```python
from build123d import *

# Parameters (mm, degrees)
BOSS_EXTRUDE3_DEPTH = 37
SKETCH7_OUTSIDE_W   = 24.466
SKETCH7_OUTSIDE_H   = 49.466
CUT_EXTRUDE4_DEPTH  = 37
SKETCH8_R           = 1.5
CUT_EXTRUDE5_DEPTH  = 3.5
SKETCH9_R           = 1.5
CUT_EXTRUDE6_DEPTH  = 3.5
SKETCH10_R          = 1.4
BOSS_EXTRUDE4_DEPTH = 3


with BuildPart() as part:
    # Sketch1 → Boss-Extrude3 (new body)
    with BuildSketch(Plane(origin=(0, 0, 0), x_dir=(1, 0, 0), z_dir=(0, 1, 0))):
        Polygon((-15.830224571, 22.390751722), (-15.830224571, -12.609248278), (-3.830224571, -12.609248278), (-3.830224571, -6.609248278), (-9.830224571, -6.609248278), (-9.830224571, 22.390751722), align=None)
    extrude(amount=BOSS_EXTRUDE3_DEPTH)

    # Sketch7 outside → Cut-Extrude4 (cut)
    with BuildSketch(Plane(origin=(0, 0, -22.390751722), x_dir=(-1, 0, 0), z_dir=(0, 0, -1))):
        with Locations((9.83, 18.5)):
            Rectangle(SKETCH7_OUTSIDE_W, SKETCH7_OUTSIDE_H)
        with BuildLine():
            Line((12.830224571, 37), (-5.541662032, 37))
            Line((-5.541662032, 37), (-5.541662032, 0))
            Line((-5.541662032, 0), (12.830224571, 0))
            ThreePointArc((12.830224571, 0), (14.951544915, 0.878679656), (15.830224571, 3))
            Line((15.830224571, 3), (15.830224571, 34))
            ThreePointArc((15.830224571, 34), (14.951544915, 36.121320344), (12.830224571, 37))
        make_face(mode=Mode.SUBTRACT)
    extrude(amount=-CUT_EXTRUDE4_DEPTH, mode=Mode.SUBTRACT)

    # Sketch8 → Cut-Extrude5 (cut)
    with BuildSketch(Plane(origin=(-9.830224571, 0, 0), x_dir=(0, 0, -1), z_dir=(1, 0, 0))):
        with Locations((-0.109248278, 34)):
            Circle(SKETCH8_R)
        with Locations((8.890751722, 34)):
            Circle(SKETCH8_R)
        with Locations((-0.109248278, 3)):
            Circle(SKETCH8_R)
        with Locations((8.890751722, 3)):
            Circle(SKETCH8_R)
        with Locations((17.890751722, 3)):
            Circle(SKETCH8_R)
        with Locations((17.890751722, 34)):
            Circle(SKETCH8_R)
    extrude(amount=-CUT_EXTRUDE5_DEPTH, mode=Mode.SUBTRACT)

    # Sketch9 → Cut-Extrude6 (cut)
    with BuildSketch(Plane(origin=(0, 0, 6.609248278), x_dir=(-1, 0, 0), z_dir=(0, 0, -1))):
        with Locations((6.830224571, 34)):
            Circle(SKETCH9_R)
        with Locations((6.830224571, 3)):
            Circle(SKETCH9_R)
    extrude(amount=-CUT_EXTRUDE6_DEPTH, mode=Mode.SUBTRACT)

    # Sketch10 → Boss-Extrude4 (add)
    with BuildSketch(Plane(origin=(-9.830224571, 0, 0), x_dir=(0, 0, -1), z_dir=(1, 0, 0))):
        with Locations(Location((4.390751722, 3, 0), (0, 0, 180))):
            Circle(SKETCH10_R)
        with Locations(Location((4.390751722, 34, 0), (0, 0, 180))):
            Circle(SKETCH10_R)
        with Locations(Location((13.390751722, 3, 0), (0, 0, 180))):
            Circle(SKETCH10_R)
        with Locations(Location((13.390751722, 34, 0), (0, 0, 180))):
            Circle(SKETCH10_R)
    extrude(amount=BOSS_EXTRUDE4_DEPTH)


solid = part.part
```
The model under review builds one solid part; all positions refer to its coordinate system, in mm. A direction names the side the tool comes from. Round coordinates to 2 decimals unless told otherwise and drop trailing zeros. Order: outer loops, then holes, each group sorted by start corner. A loop starts at its lowest first (then second) coordinate and runs counter-clockwise, first axis right, second up. Notation, with made-up numbers: (-10, 27.25) -> (24, 27.25) arc R6 ccw to (24, 38.25) -> close; hole circle Ø11 at (-4.75, 37). An arc over 180 degrees is marked (long way). One line per item, written item: value. Start each with the question number.
Q1. Machinability: for faces 1 (the face through (-6.83, 34, -13)), 2 (the face through (-7, 3, 10.109)), 3 (the face through (-14.93, 0.86, -5.14)), 4 (the face through (-11.56, 33.09, -16.7)), which of the approach directions +Z, -Z, +X, -X, +Y, -Y give a long, thin tool a straight path to every point of the face, cutting with its end or side? Answer none if there is none.
Q2. Take a section at C-C (x = -6.25). Write out the cut boundary in (y, z).
Q3. Take a section at D-D (z = -14). Write out the cut boundary in (x, y).
Q4. Wall thickness on line 1 (X direction, y = 34, z = -0.5); line 2 (X direction, y = 21.5, z = -11.5); line 3 (Z direction, x = -6.25, y = 35): over which ranges is each line inside the solid? List them lowest first.
Q5. Clearance check with flat-ended pins moving along their axes: pin 1 Ø2.5 at (y, z) = (3, -9) entering from +X; pin 2 Ø2 at (y, z) = (21.5, 5.5) entering from +X; pin 3 Ø1.5 at (x, y) = (-6.5, 3) entering from -Z. State where each tip first meets the part, or that it passes through.
Q6. Take a section at B-B (z = -2). Write out the cut boundary in (x, y).
Q7. Take a section at A-A (y = 12.5). Write out the cut boundary in (x, z), and give its area (3 significant figures).
Q8. Mouldability with a two-part tool opening along Y and no side actions: class faces 5 (the face through (-6.83, 3, -13)), 6 (the face through (-13.33, 34, -9)), 7 (the face through (-10, 37, -1)) as released by +Y, released by -Y, zero draft, split by the parting line, or undercut.
Reported:
1. face 1: -Z, +X, +Y, -Y
1. face 2: none
1. face 3: +Z, -Z, -X, -Y
1. face 4: +X
2. outline: (0, 6.61) -> (1.62, 6.61) -> (1.62, 10.11) -> (4.38, 10.11) -> (4.38, 6.61) -> (32.62, 6.61) -> (32.62, 10.11) -> (35.38, 10.11) -> (35.38, 6.61) -> (37, 6.61) -> (37, 12.61) -> (0, 12.61) -> close
3. outline: (-15.83, 3) arc R3 ccw to (-12.83, 0) -> (-9.83, 0) -> (-9.83, 1.74) -> (-6.83, 1.74) -> (-6.83, 4.26) -> (-9.83, 4.26) -> (-9.83, 32.74) -> (-6.83, 32.74) -> (-6.83, 35.26) -> (-9.83, 35.26) -> (-9.83, 37) -> (-12.83, 37) arc R3 ccw to (-15.83, 34) -> close
4. line 1: x = -15.83 to -13.33
4. line 2: x = -15.83 to -9.83
4. line 3: z = 10.11 to 12.61
5. pin 1: stops at x = -13.33
5. pin 2: stops at x = -9.83
5. pin 3: stops at z = -14.79
6. outline: (-15.83, 3) arc R3 ccw to (-12.83, 0) -> (-9.83, 0) -> (-9.83, 37) -> (-12.83, 37) arc R3 ccw to (-15.83, 34) -> close
7. outline: (-15.83, -22.39) -> (-9.83, -22.39) -> (-9.83, 6.61) -> (-3.83, 6.61) -> (-3.83, 12.61) -> (-15.83, 12.61) -> close
7. area: 246 mm2
8. face 5: zero draft
8. face 6: undercut
8. face 7: released by +Y
